```python
from build123d import *

# Parameters (mm, degrees)
ESBO_O1_W                = 90
ESBO_O1_H                = 70
RESSALTO_EXTRUS_O1_DEPTH = 2
ESBO_O3_W                = 4
ESBO_O3_H                = 9
ESBO_O3_W_2              = 9
ESBO_O3_H_2              = 4
RESSALTO_EXTRUS_O4_DEPTH = 8
ESBO_O6_W                = 66
ESBO_O6_H                = 15
CORTE_EXTRUS_O4_DEPTH    = 3
ESBO_O7_R                = 1.6
CORTE_EXTRUS_O7_DEPTH    = 3
ESBO_O8_R                = 1.6
CORTE_EXTRUS_O8_DEPTH    = 5
ESBO_O9_R                = 1.6
CORTE_EXTRUS_O9_DEPTH    = 5
ESBO_O10_R               = 1.6
CORTE_EXTRUS_O10_DEPTH   = 5
ESBO_O11_R               = 1.6
CORTE_EXTRUS_O11_DEPTH   = 5
ESBO_O12_R               = 1.6
CORTE_EXTRUS_O12_DEPTH   = 58.567351858
ESBO_O2_W                = 5.334
ESBO_O2_H                = 5.45
CORTE_EXTRUS_O13_DEPTH   = 58.567351858


with BuildPart() as part:
    # Esboço1 → Ressalto-extrusão1 (new body)
    with BuildSketch(Plane(origin=(0, 0, 0), x_dir=(1, 0, 0), z_dir=(0, 1, 0))):
        Rectangle(ESBO_O1_W, ESBO_O1_H)
    extrude(amount=RESSALTO_EXTRUS_O1_DEPTH)

    # Esboço3 → Ressalto-extrusão4 (add)
    with BuildSketch(Plane(origin=(0, 2, 0), x_dir=(1, 0, 0), z_dir=(0, 1, 0))):
        with Locations((-38, 30.5)):
            Rectangle(ESBO_O3_W, ESBO_O3_H)
        with Locations((40.5, 28)):
            Rectangle(ESBO_O3_W_2, ESBO_O3_H_2)
        with Locations((38, -30.5)):
            Rectangle(ESBO_O3_W, ESBO_O3_H)
        with Locations((-40.5, -28)):
            Rectangle(ESBO_O3_W_2, ESBO_O3_H_2)
    extrude(amount=RESSALTO_EXTRUS_O4_DEPTH)

    # Esboço6 → Corte-extrusão4 (cut)
    with BuildSketch(Plane.XZ):
        with Locations((0, -22.5)):
            Rectangle(ESBO_O6_W, ESBO_O6_H)
    extrude(amount=-CORTE_EXTRUS_O4_DEPTH, mode=Mode.SUBTRACT)

    # Esboço7 → Corte-extrusão7 (cut)
    with BuildSketch(Plane(origin=(0, 2, 0), x_dir=(1, 0, 0), z_dir=(0, 1, 0))):
        with Locations(Location((31.5, 9, 0), (0, 0, 270))):
            Circle(ESBO_O7_R)
        with Locations(Location((-5.5, 9, 0), (0, 0, 270))):
            Circle(ESBO_O7_R)
        with Locations(Location((-5.5, -28, 0), (0, 0, 270))):
            Circle(ESBO_O7_R)
        with Locations(Location((31.5, -28, 0), (0, 0, 270))):
            Circle(ESBO_O7_R)
    extrude(amount=-CORTE_EXTRUS_O7_DEPTH, mode=Mode.SUBTRACT)

    # Esboço8 → Corte-extrusão8 (cut)
    with BuildSketch(Plane(origin=(0, 0, -30), x_dir=(-1, 0, 0), z_dir=(0, 0, -1))):
        with Locations((-40.5, 6)):
            Circle(ESBO_O8_R)
    extrude(amount=-CORTE_EXTRUS_O8_DEPTH, mode=Mode.SUBTRACT)

    # Esboço9 → Corte-extrusão9 (cut)
    with BuildSketch(Plane.ZY.offset(40)):
        with Locations((-30.5, 6)):
            Circle(ESBO_O9_R)
    extrude(amount=-CORTE_EXTRUS_O9_DEPTH, mode=Mode.SUBTRACT)

    # Esboço10 → Corte-extrusão10 (cut)
    with BuildSketch(Plane.XY.offset(30)):
        with Locations((-40.5, 6)):
            Circle(ESBO_O10_R)
    extrude(amount=-CORTE_EXTRUS_O10_DEPTH, mode=Mode.SUBTRACT)

    # Esboço11 → Corte-extrusão11 (cut)
    with BuildSketch(Plane(origin=(40, 0, 0), x_dir=(0, 0, -1), z_dir=(1, 0, 0))):
        with Locations((-30.5, 6)):
            Circle(ESBO_O11_R)
    extrude(amount=-CORTE_EXTRUS_O11_DEPTH, mode=Mode.SUBTRACT)

    # Esboço12 → Corte-extrusão12 (cut, through all)
    with BuildSketch(Plane(origin=(0, 2, 0), x_dir=(1, 0, 0), z_dir=(0, 1, 0))):
        with Locations(Location((-40.5, 22.5, 0), (0, 0, 270))):
            Circle(ESBO_O12_R)
        with Locations(Location((-40.5, -22.5, 0), (0, 0, 270))):
            Circle(ESBO_O12_R)
        with Locations(Location((40.5, -22.5, 0), (0, 0, 270))):
            Circle(ESBO_O12_R)
        with Locations(Location((40.5, 22.5, 0), (0, 0, 270))):
            Circle(ESBO_O12_R)
    extrude(amount=-CORTE_EXTRUS_O12_DEPTH, mode=Mode.SUBTRACT)

    # Esboço2 → Corte-extrusão13 (cut, through all)
    with BuildSketch(Plane(origin=(0, 2, 0), x_dir=(1, 0, 0), z_dir=(0, 1, 0))):
        with Locations((-26.663, -5.455)):
            Rectangle(ESBO_O2_W, ESBO_O2_H)
        with Locations((-15.993, -5.455)):
            Rectangle(ESBO_O2_W, ESBO_O2_H)
        with Locations((-5.323, -5.455)):
            Rectangle(ESBO_O2_W, ESBO_O2_H)
        with Locations((5.347, -5.455)):
            Rectangle(ESBO_O2_W, ESBO_O2_H)
        with Locations((16.017, -5.455)):
            Rectangle(ESBO_O2_W, ESBO_O2_H)
        with Locations((26.687, -5.455)):
            Rectangle(ESBO_O2_W, ESBO_O2_H)
        with Locations((37.357, -5.455)):
            Rectangle(ESBO_O2_W, ESBO_O2_H)
        with Locations((-26.663, -16.365)):
            Rectangle(ESBO_O2_W, ESBO_O2_H)
        with Locations((-15.993, -16.365)):
            Rectangle(ESBO_O2_W, ESBO_O2_H)
        with Locations((-5.323, -16.365)):
            Rectangle(ESBO_O2_W, ESBO_O2_H)
        with Locations((5.347, -16.365)):
            Rectangle(ESBO_O2_W, ESBO_O2_H)
        with Locations((16.017, -16.365)):
            Rectangle(ESBO_O2_W, ESBO_O2_H)
        with Locations((26.687, -16.365)):
            Rectangle(ESBO_O2_W, ESBO_O2_H)
        with Locations((-37.333, -5.455)):
            Rectangle(ESBO_O2_W, ESBO_O2_H)
    extrude(amount=-CORTE_EXTRUS_O13_DEPTH, mode=Mode.SUBTRACT)


solid = part.part
```
The model under review builds one solid part; all positions refer to its coordinate system, in mm. A direction names the side the tool comes from. Round coordinates to 2 decimals unless told otherwise and drop trailing zeros. Loops run counter-clockwise (first coordinate to the right, second up) from the corner with the lowest first, then second, coordinate; pieces in that order, holes last. Notation, with made-up numbers: (86, 75) -> (93, 75) arc R12 cw to (93, 98) -> close; hole circle Ø1 at (68.5, 75). An arc over 180 degrees is marked (long way). Answer as a JSON object with one key per item and string values. Group by question number.
1) We need section C-C on z = -9. Write out the cut boundary in (x, y), then the cut area to 3 significant figures.
2) For pin 1 Ø6 at (y, z) = (5.5, -14) entering from -X; pin 2 Ø1 at (x, z) = (-7.5, 12.5) entering from +Y; pin 3 Ø2.5 at (y, z) = (7.5, -32) entering from -X; pin 4 Ø4 at (x, y) = (42.5, 5) entering from +Z, all flat-tipped, find the tip position at first contact; note any pin that passes through.
3) We need section D-D on z = -22.5. Write out the cut boundary in (x, y).
4) We need section B-B on y = 6. Give the number of separate pieces and of enclosed holes in the cut face, then the cut area to 3 significant figures.
5) Mouldability with a two-part tool opening along Z and no side actions: class faces 1 (the face through (27, 1, 2.73)), 2 (the face through (38, 10, 30)) as released by +Z, released by -Z, zero draft, split by the parting line, or undercut.
6) For line 1 (X direction, y = 0.5, z = -22.5); line 2 (Y direction, x = 40.5, z = -27.8); line 3 (X direction, y = 8.5, z = -28), list the stretches that pass through material, from the lowest coordinate up. Write a range as [from, to].
7) For faces 3 (the face through (-36, 4, -30)), 4 (the face through (33, 1, -23)), 5 (the face through (-40.85, 4.44, 28.03)), list the 3-axis set-ups (+Z, -Z, +X, -X, +Y, -Y) from which the entire face can be reached by the end or side of a thin tool; tool diameter is ignored.
8) We need section A-A on z = 18. Write out the cut boundary in (x, y), then the cut area to 3 significant figures.
Result set:
{
 "1": {"outline": "(-45, 0) -> (-7.1, 0) -> (-7.1, 2) -> (-45, 2) -> close; (-3.9, 0) -> (29.9, 0) -> (29.9, 2) -> (-3.9, 2) -> close; (33.1, 0) -> (45, 0) -> (45, 2) -> (33.1, 2) -> close", "area": "167 mm²"},
 "2": {"pin 1": "through", "pin 2": "y = 2", "pin 3": "x = -40", "pin 4": "z = -26"},
 "3": {"outline": "(-45, 0) -> (-42.1, 0) -> (-42.1, 2) -> (-45, 2) -> close; (-38.9, 0) -> (-33, 0) -> (-33, 2) -> (-38.9, 2) -> close; (33, 0) -> (38.9, 0) -> (38.9, 2) -> (33, 2) -> close; (42.1, 0) -> (45, 0) -> (45, 2) -> (42.1, 2) -> close"},
 "4": {"separate pieces": "8", "enclosed holes": "0", "area": "92.8 mm²"},
 "5": {"face 1": "undercut", "face 2": "zero draft"},
 "6": {"line 1": "[-45, -42.1], [-38.9, -33], [33, 38.9], [42.1, 45]", "line 2": "[0, 4.4], [7.6, 10]", "line 3": "[-40, -36], [36, 45]"},
 "7": {"face 3": "+Z, -Z, +Y", "face 4": "+Y, -Y", "face 5": "+Z"},
 "8": {"outline": "(-45, 0) -> (-29.33, 0) -> (-29.33, 2) -> (-45, 2) -> close; (-24, 0) -> (-18.66, 0) -> (-18.66, 2) -> (-24, 2) -> close; (-13.33, 0) -> (-7.99, 0) -> (-7.99, 2) -> (-13.33, 2) -> close; (-2.66, 0) -> (2.68, 0) -> (2.68, 2) -> (-2.66, 2) -> close; (8.01, 0) -> (13.35, 0) -> (13.35, 2) -> (8.01, 2) -> close; (18.68, 0) -> (24.02, 0) -> (24.02, 2) -> (18.68, 2) -> close; (29.35, 0) -> (45, 0) -> (45, 2) -> (29.35, 2) -> close", "area": "116 mm²"}
}
